```python
from build123d import *

# Parameters (mm, degrees)
SKETCH_1_W          = 140
SKETCH_1_H          = 75
EXTRUDE_1_DEPTH     = 61
SHELL_1_T           = -1.5
SKETCH_3_W          = 130
SKETCH_3_H          = 65
CUT_EXTRUDE_1_DEPTH = 117.308601118
SKETCH_4_W          = 137
SKETCH_4_H          = 2.6
SKETCH_4_H_2        = 3.3
EXTRUDE_2_DEPTH     = 5
SKETCH_5_W          = 2.4
SKETCH_5_H          = 69.4
EXTRUDE_3_DEPTH     = 5
SKETCH_29_W         = 2
SKETCH_29_H         = 29.319547491
EXTRUDE_4_DEPTH     = 2


# Read off the part's stored shape, not the designer's step: M3 六角凹锥坑螺钉的锥形沉头孔1, M3 六角凹锥坑螺钉的锥形沉头孔2
with BuildPart() as part:
    # 草图1 → 凸台-拉伸1 (new body)
    with BuildSketch(Plane.XY):
        with Locations((19.248188406, -5.412137681)):
            Rectangle(SKETCH_1_W, SKETCH_1_H)
    extrude(amount=EXTRUDE_1_DEPTH)

    # 抽壳1
    shell_1_openings = [part.faces().sort_by_distance(p)[0] for p in [
        (19.248188406, -5.412137681, 61),
    ]]
    offset(amount=SHELL_1_T, openings=shell_1_openings, kind=Kind.INTERSECTION)

    # 草图3 → 切除-拉伸1 (cut, through all)
    with BuildSketch(Plane(origin=(0, 0, 0), x_dir=(-1, 0, 0), z_dir=(0, 0, -1))):
        with Locations((-19.248188406, -5.412137681)):
            Rectangle(SKETCH_3_W, SKETCH_3_H)
    extrude(amount=-CUT_EXTRUDE_1_DEPTH, mode=Mode.SUBTRACT)

    # 草图4 → 凸台-拉伸2 (add)
    with BuildSketch(Plane.XY.offset(1.5)):
        with Locations((19.248188406, -40.112137681)):
            Rectangle(SKETCH_4_W, SKETCH_4_H)
        with Locations((19.248188406, 28.937862319)):
            Rectangle(SKETCH_4_W, SKETCH_4_H_2)
    extrude(amount=EXTRUDE_2_DEPTH)

    # 草图5 → 凸台-拉伸3 (add)
    with BuildSketch(Plane.XY.offset(1.5)):
        with Locations((-48.051811594, -4.112137681)):
            Rectangle(SKETCH_5_W, SKETCH_5_H)
        with Locations((86.548188406, -4.112137681)):
            Rectangle(SKETCH_5_W, SKETCH_5_H)
    extrude(amount=EXTRUDE_3_DEPTH)

    # M3 六角凹锥坑螺钉的锥形沉头孔1 outline → M3 六角凹锥坑螺钉的锥形沉头孔1 (revolve, cut)
    with BuildSketch(Plane(origin=(0, -28.118319618, 54.934676649), x_dir=(0, 1, 0), z_dir=(0, 0, -1))):
        Polygon((0, -50.751811594), (3.36, -50.751811594), (1.86, -49.251811594), (0, -49.251811594), align=None)
    revolve(axis=Axis((0, -28.118319618, 54.934676649), (1, 0, 0)), mode=Mode.SUBTRACT)

    # Hole Wizard M3 _1 2 outline → Hole Wizard M3 _1 2 (revolve, cut)
    with BuildSketch(Plane(origin=(0, 21.583463225, 54.934676649), x_dir=(0, 1, 0), z_dir=(0, 0, -1))):
        Polygon((0, -50.751811594), (3.36, -50.751811594), (1.86, -49.251811594), (0, -49.251811594), align=None)
    revolve(axis=Axis((0, 21.583463225, 54.934676649), (1, 0, 0)), mode=Mode.SUBTRACT)

    # M3 六角凹锥坑螺钉的锥形沉头孔2 outline → M3 六角凹锥坑螺钉的锥形沉头孔2 (revolve, cut)
    with BuildSketch(Plane(origin=(0, -28.118319618, 54.934676649), x_dir=(0, 1, 0), z_dir=(0, 0, -1))):
        Polygon((3.36, 89.248188406), (0, 89.248188406), (0, 87.748188406), (1.86, 87.748188406), align=None)
    revolve(axis=Axis((0, -28.118319618, 54.934676649), (1, 0, 0)), mode=Mode.SUBTRACT)

    # Hole Wizard M3 _2 2 outline → Hole Wizard M3 _2 2 (revolve, cut)
    with BuildSketch(Plane(origin=(0, 21.583463225, 54.934676649), x_dir=(0, 1, 0), z_dir=(0, 0, -1))):
        Polygon((3.36, 89.248188406), (0, 89.248188406), (0, 87.748188406), (1.86, 87.748188406), align=None)
    revolve(axis=Axis((0, 21.583463225, 54.934676649), (1, 0, 0)), mode=Mode.SUBTRACT)

    # 草图29 → 凸台-拉伸4 (add)
    with BuildSketch(Plane(origin=(0, -41.412137681, 0), x_dir=(1, 0, 0), z_dir=(0, 1, 0))):
        with Locations((35.5, -33.722670624)):
            Rectangle(SKETCH_29_W, SKETCH_29_H)
        with Locations((66, -33.722670624)):
            Rectangle(SKETCH_29_W, SKETCH_29_H)
    extrude(amount=EXTRUDE_4_DEPTH)


solid = part.part
```
Model file for the job. Use its own axes, mm. A direction names the side the tool comes from. Give positions to 0.01 mm unless a question says otherwise; leave off trailing zeros. Order: outer loops, then holes, each group sorted by start corner. A loop starts at its lowest first (then second) coordinate and runs counter-clockwise, first axis right, second up.
1) Saw through at A-A, the plane y = -11.5. Write the cut outline in (x, z), then the cut area to 4 significant figures.
2) Saw through at D-D, the plane y = 20. Count the separate pieces of the cut face and the enclosed holes in it, then the cut area to 3 significant figures.
3) Wall check: probe 1 along Y at (x, z) = (78, 28); probe 2 along X at (y, z) = (-25, 47); probe 3 along Y at (x, z) = (27.5, 3.5). Give the ranges that are in metal, low to high.
4) 3-axis set-ups, long thin cutter, end or side, ignore diameter. For faces 5 (the flat face through (18, -42.912, 30)), 6 (the flat face through (18, 30.588, 33)): which of +Z, -Z, +X, -X, +Y, -Y reach the whole face in a straight line?
5) Pin check, flat tip, straight feed: pin 1 (6 mm diameter, centred on x = -29, y = -35, fed in from +Z). Stop position of the tip, or through.
6) Saw through at C-C, the plane z = 37. Write the cut outline in (x, y).
7) Saw through at B-B, the plane x = 48. Write the cut outline in (y, z).
8) Mould opens along X. For faces 1 (the flat face through (14, -39, 0)), 2 (the flat face through (89.248, -6, 30)), 3 (the flat face through (18, -38.812, 4)), 4 (the flat face through (-46.852, -6, 4)) say: +X half, -X half, draft (parallel to the pull), parting line (faces both ways), or undercut.
Computed:
1. outline: (-50.75, 0) - (-45.75, 0) - (-45.75, 1.5) - (-46.85, 1.5) - (-46.85, 6.5) - (-49.25, 6.5) - (-49.25, 61) - (-50.75, 61) - close; (84.25, 0) - (89.25, 0) - (89.25, 61) - (87.75, 61) - (87.75, 6.5) - (85.35, 6.5) - (85.35, 1.5) - (84.25, 1.5) - close
1. area: 217.5 mm2
2. separate pieces: 4
2. enclosed holes: 0
2. area: 205 mm2
3. probe 1: y = -42.91 to -41.41, 30.59 to 32.09
3. probe 2: x = -50.75 to -49.25, 87.75 to 89.25
3. probe 3: y = -42.91 to -38.81, 27.29 to 32.09
4. face 5: +Z, -Z, +X, -X, -Y
4. face 6: +Z
5. pin 1: stops at z = 1.5
6. outline: (-50.75, -42.91) - (89.25, -42.91) - (89.25, 32.09) - (-50.75, 32.09) - close; hole (-49.25, -41.41) - (34.5, -41.41) - (34.5, -39.41) - (36.5, -39.41) - (36.5, -41.41) - (65, -41.41) - (65, -39.41) - (67, -39.41) - (67, -41.41) - (87.75, -41.41) - (87.75, 30.59) - (-49.25, 30.59) - close
7. outline: (-42.91, 0) - (-37.91, 0) - (-37.91, 1.5) - (-38.81, 1.5) - (-38.81, 6.5) - (-41.41, 6.5) - (-41.41, 61) - (-42.91, 61) - close; (27.09, 0) - (32.09, 0) - (32.09, 61) - (30.59, 61) - (30.59, 6.5) - (27.29, 6.5) - (27.29, 1.5) - (27.09, 1.5) - close
8. face 1: draft
8. face 2: +X half
8. face 3: undercut
8. face 4: undercut
